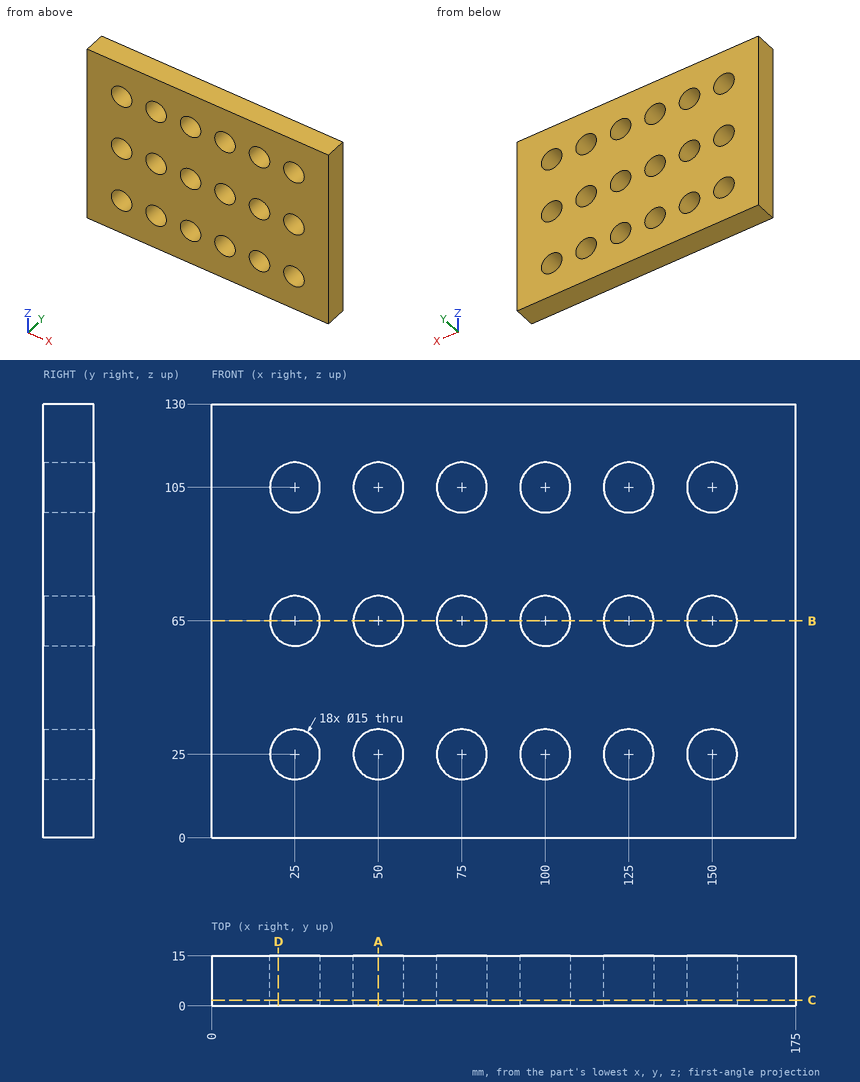
Geometry check sheet. Reference: drawing and pictorial views, mm from the part's lowest x, y, z. Give positions to 0.01 mm unless a question says otherwise; leave off trailing zeros. Order: outer loops, then holes, each group sorted by start corner. A loop starts at its lowest first (then second) coordinate and runs counter-clockwise, first axis right, second up. Notation, with made-up numbers: M -13,82 L 19,82 A7 ccw 19,88 Z; hole C -11.75,47.5 d3. An arc over 180 degrees is marked long. Answer as a JSON object with one key per item and string values. Group by question number.
1) Cross-section at D-D (x = 20). Enter the section's corners in (y, z), then the cut area to 3 significant figures.
2) Cross-section at B-B (z = 65). Enter the section's corners in (x, y).
3) Cross-section at A-A (x = 50). Enter the section's corners in (y, z).
4) Scan lines: line 1 along Z through (x, y) = (50, 11); line 2 along Z through (x, y) = (69.5, 0.75). Record each from-to range of solid material in increasing order. Write a range as [from, to].
5) Cross-section at C-C (y = 1.75). Give the number of separate pieces and of enclosed holes in the cut face, then the cut area to 3 significant figures.
Result sheet:
{
 "1": {"outline": "M 0,0 L 15,0 L 15,19.41 L 0,19.41 Z; M 0,30.59 L 15,30.59 L 15,59.41 L 0,59.41 Z; M 0,70.59 L 15,70.59 L 15,99.41 L 0,99.41 Z; M 0,110.59 L 15,110.59 L 15,130 L 0,130 Z", "area": "1,450 mm2"},
 "2": {"outline": "M 0,0 L 17.5,0 L 17.5,15 L 0,15 Z; M 32.5,0 L 42.5,0 L 42.5,15 L 32.5,15 Z; M 57.5,0 L 67.5,0 L 67.5,15 L 57.5,15 Z; M 82.5,0 L 92.5,0 L 92.5,15 L 82.5,15 Z; M 107.5,0 L 117.5,0 L 117.5,15 L 107.5,15 Z; M 132.5,0 L 142.5,0 L 142.5,15 L 132.5,15 Z; M 157.5,0 L 175,0 L 175,15 L 157.5,15 Z"},
 "3": {"outline": "M 0,0 L 15,0 L 15,17.5 L 0,17.5 Z; M 0,32.5 L 15,32.5 L 15,57.5 L 0,57.5 Z; M 0,72.5 L 15,72.5 L 15,97.5 L 0,97.5 Z; M 0,112.5 L 15,112.5 L 15,130 L 0,130 Z"},
 "4": {"line 1": "z = [0, 17.5], [32.5, 57.5], [72.5, 97.5], [112.5, 130]", "line 2": "z = [0, 19.9], [30.1, 59.9], [70.1, 99.9], [110.1, 130]"},
 "5": {"separate pieces": "1", "enclosed holes": "18", "area": "19,600 mm2"}
}
